Verification items for the finished model (mm, model axes). Coordinates: 2 decimals unless noted, no trailing zeros. Loops run counter-clockwise (first coordinate to the right, second up) from the corner with the lowest first, then second, coordinate; pieces in that order, holes last. Notation, with made-up numbers: (-2, 28) - (47, 28) arc R29 ccw to (47, 53) - close; hole circle Ø5 at (52.5, 8). An arc over 180 degrees is marked (long way). One line per item, written item: value. Start each with the question number.
(1) Gauge pin test, flat ends, axial feed: P1, Ø5, axis at x = -18, y = -14.5, coming from the +Z side (3 decimals); P2, Ø1, axis at y = -68, z = 1, coming from the +X side (3 decimals); P3, Ø1, axis at y = -29, z = 2, coming from the +X side; P4, Ø1.6, axis at x = -14, z = 2, coming from the -Y side. Record the tip position at first contact, or that the pin passes through.
(2) Thickness scan on probe 1 along X at (y, z) = (-32.5, 1.5); probe 2 along Y at (x, z) = (-32, 0.8); probe 3 along Y at (x, z) = (-7.5, 2.7). Record the ranges inside material, lowest first. Write a range as [from, to].
(3) Section check B-B (y = -15). Record the boundary of the cut face in (x, z) (3 decimals), plus the area to 3 significant figures.
(4) Section check C-C (x = 2). Record the boundary of the cut face in (y, z) (3 decimals), plus the area to 3 significant figures.
(5) Section check A-A (z = 2.6). Record the boundary of the cut face in (x, y) (3 decimals), plus the area to 3 significant figures.
```python
from build123d import *

# Parameters (mm, degrees)
SKETCH1_W           = 12.7
SKETCH1_H           = 12.7
BOSS_EXTRUDE1_DEPTH = 3.175
CUT_EXTRUDE1_DEPTH  = 4.175
SKETCH4_W           = 3.175
SKETCH4_H           = 6.35
BOSS_EXTRUDE3_DEPTH = 3.175
SKETCH5_W           = 3.175
SKETCH5_H           = 12.7
BOSS_EXTRUDE4_DEPTH = 41.91
SKETCH6_W           = 12.7
SKETCH6_H           = 3.175
BOSS_EXTRUDE5_DEPTH = 53.34
SKETCH7_W           = 6.35
SKETCH7_H           = 3.175
BOSS_EXTRUDE6_DEPTH = 3.175


with BuildPart() as part:
    # Sketch1 → Boss-Extrude1 (new body)
    with BuildSketch(Plane.XY):
        with Locations((6.35, -6.35)):
            Rectangle(SKETCH1_W, SKETCH1_H)
    extrude(amount=BOSS_EXTRUDE1_DEPTH)

    # Sketch3 → Cut-Extrude1 (cut, through all)
    with BuildSketch(Plane(origin=(0, 0, 0), x_dir=(-1, 0, 0), z_dir=(0, 0, -1))):
        Polygon((0, 0), (-12.7, -12.7), (-12.7, 0), align=None)
    extrude(amount=-CUT_EXTRUDE1_DEPTH, mode=Mode.SUBTRACT)

    # Sketch4 → Boss-Extrude3 (add)
    with BuildSketch(Plane(origin=(0, 0, 0), x_dir=(0, 0, -1), z_dir=(0.707106781, 0.707106781, 0))):
        with Locations((-1.5875, -8.980256121)):
            Rectangle(SKETCH4_W, SKETCH4_H)
    extrude(amount=BOSS_EXTRUDE3_DEPTH)

    # Sketch5 → Boss-Extrude4 (add)
    with BuildSketch(Plane.ZY):
        with Locations((1.5875, -6.35)):
            Rectangle(SKETCH5_W, SKETCH5_H)
    extrude(amount=BOSS_EXTRUDE4_DEPTH)

    # Sketch6 → Boss-Extrude5 (add)
    with BuildSketch(Plane(origin=(0, -12.7, 0), x_dir=(-1, 0, 0), z_dir=(0, -1, 0))):
        with Locations((35.56, -1.5875)):
            Rectangle(SKETCH6_W, SKETCH6_H)
    extrude(amount=BOSS_EXTRUDE5_DEPTH)

    # Sketch7 → Boss-Extrude6 (add)
    with BuildSketch(Plane.XZ.offset(66.04)):
        with Locations((-35.56, 1.5875)):
            Rectangle(SKETCH7_W, SKETCH7_H)
    extrude(amount=BOSS_EXTRUDE6_DEPTH)


solid = part.part
```
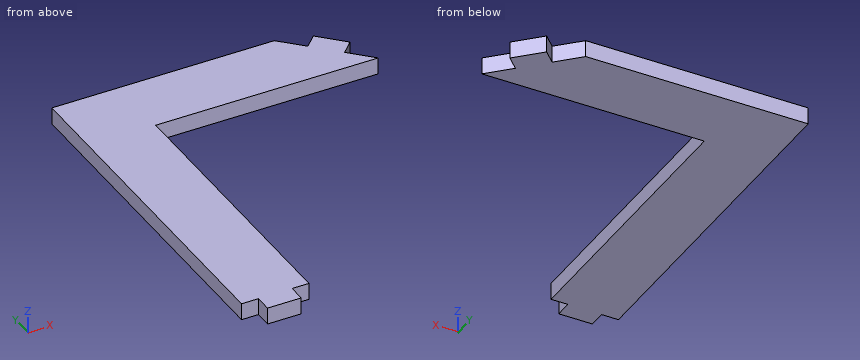
Responses:
1. P1: stops at z = 3.175
1. P2: stops at x = -32.385
1. P3: stops at x = -29.21
1. P4: stops at y = -12.7
2. probe 1: x = [-41.91, -29.21]
2. probe 2: y = [-66.04, 0]
2. probe 3: y = [-12.7, 0]
3. outline: (-41.91, 0) - (-29.21, 0) - (-29.21, 3.175) - (-41.91, 3.175) - close
3. area: 40.3 mm²
4. outline: (-12.7, 0) - (-2, 0) - (-2, 3.175) - (-12.7, 3.175) - close
4. area: 34.0 mm²
5. outline: (-41.91, -66.04) - (-38.735, -66.04) - (-38.735, -69.215) - (-32.385, -69.215) - (-32.385, -66.04) - (-29.21, -66.04) - (-29.21, -12.7) - (12.7, -12.7) - (8.595, -8.595) - (10.84, -6.35) - (6.35, -1.86) - (4.105, -4.105) - (0, 0) - (-41.91, 0) - close
5. area: 1,330 mm²
